from build123d import *

# Parameters (mm, degrees)
SKETCH002_W  = 7.7
SKETCH002_H  = 9.35
PAD_DEPTH    = 1
SKETCH003_W  = 7.7
SKETCH003_H  = 9.35
PAD001_DEPTH = 2.5
SKETCH004_W  = 7.7
SKETCH004_H  = 9.35
PAD002_DEPTH = 1.8
SKETCH005_R  = 3.5
PAD003_DEPTH = 5
SKETCH006_R  = 3.000001
PAD004_DEPTH = 3
PAD005_DEPTH = 7


with BuildPart() as part:
    # Sketch002 (on DatumPlane) → Pad (new body)
    with BuildSketch(Plane.XY):
        with Locations((0, -0.825)):
            Rectangle(SKETCH002_W, SKETCH002_H)
    extrude(amount=PAD_DEPTH)

    # Sketch003 (on DatumPlane) → Pad001 (join)
    with BuildSketch(Plane.XY.offset(1)):
        with Locations((0, -0.825)):
            Rectangle(SKETCH003_W, SKETCH003_H)
    extrude(amount=PAD001_DEPTH)

    # Sketch004 (on DatumPlane) → Pad002 (join)
    with BuildSketch(Plane.XY.offset(3.5)):
        with Locations((0, -0.825)):
            Rectangle(SKETCH004_W, SKETCH004_H)
    extrude(amount=PAD002_DEPTH)

    # Sketch005 (on DatumPlane) → Pad003 (join)
    with BuildSketch(Plane.XY.offset(5.3)):
        Circle(SKETCH005_R)
    extrude(amount=PAD003_DEPTH)

    # Sketch006 (on DatumPlane) → Pad004 (join)
    with BuildSketch(Plane.XY.offset(10.3)):
        Circle(SKETCH006_R)
    extrude(amount=PAD004_DEPTH)

    # Sketch007 (on DatumPlane) → Pad005 (join)
    with BuildSketch(Plane.XY.offset(13.3)):
        with BuildLine():
            ThreePointArc((-1.500001, 2.598077), (-1.500001, -2.598077), (3.000001, -1e-06))
            Line((-1.500001, 2.598077), (3.000001, -1e-06))
        make_face()
    extrude(amount=PAD005_DEPTH)


solid = part.part
For this review, take the finished solid that the model builds, in its own axes (mm). A direction names the side the tool comes from. Coordinates: 2 decimals unless noted, no trailing zeros. Loops run counter-clockwise (first coordinate to the right, second up) from the corner with the lowest first, then second, coordinate; pieces in that order, holes last. Notation, with made-up numbers: (48, 70) - (105, 70) arc R23 cw to (105, 90) - close; hole circle Ø10 at (63.25, -20). An arc over 180 degrees is marked (long way). Return JSON: item names as keys, results as strings.
Item 1: Take a section at D-D (y = -0.5). Give the boundary of the cut face in (x, z).
Determined:
{"outline": "(-3.85, 0) - (3.85, 0) - (3.85, 5.3) - (3.46, 5.3) - (3.46, 10.3) - (2.96, 10.3) - (2.96, 20.3) - (-2.96, 20.3) - (-2.96, 10.3) - (-3.46, 10.3) - (-3.46, 5.3) - (-3.85, 5.3) - close"}
Item 2: For line 1 (Z direction, x = 3.25, y = 0.5); line 2 (Z direction, x = -0.75, y = -4.25); line 3 (Y direction, x = -2, z = 19), list the stretches that pass through material, from the lowest coordinate up.
Determined:
{"line 1": "z = 0 to 10.3", "line 2": "z = 0 to 5.3", "line 3": "y = -2.24 to 2.24"}
Item 3: Take a section at B-B (z = 10). Give the boundary of the cut face in (x, y).
Determined:
{"outline": "circle Ø7 at (0, 0)"}
Item 4: For faces 1 (the flat face through (0.718, 1.317, 16.751)), 2 (the flat face through (3, 1, 10.3)), 3 (the flat face through (3.85, -1, 3)), list the 3-axis set-ups (+Z, -Z, +X, -X, +Y, -Y) from which the entire face can be reached by the end or side of a thin tool; tool diameter is ignored.
Determined:
{"face 1": "+Z, +X, +Y", "face 2": "+Z", "face 3": "+Z, -Z, +X, +Y, -Y"}
Item 5: Take a section at C-C (x = -1). Give the boundary of the cut face in (y, z), then the cut area to 3 significant figures.
Determined:
{"outline": "(-5.5, 0) - (3.85, 0) - (3.85, 5.3) - (3.35, 5.3) - (3.35, 10.3) - (2.83, 10.3) - (2.83, 13.3) - (2.31, 13.3) - (2.31, 20.3) - (-2.83, 20.3) - (-2.83, 10.3) - (-3.35, 10.3) - (-3.35, 5.3) - (-5.5, 5.3) - close", "area": "136 mm2"}
Item 6: Take a section at A-A (y = 0.5). Give the boundary of the cut face in (x, z), then the cut area to 3 significant figures.
Determined:
{"outline": "(-3.85, 0) - (3.85, 0) - (3.85, 5.3) - (3.46, 5.3) - (3.46, 10.3) - (2.96, 10.3) - (2.96, 13.3) - (2.13, 13.3) - (2.13, 20.3) - (-2.96, 20.3) - (-2.96, 10.3) - (-3.46, 10.3) - (-3.46, 5.3) - (-3.85, 5.3) - close", "area": "129 mm2"}
Item 7: Insertion check: pin 1 (1.5 mm diameter, centred on y = -3, z = 17, fed in from +X); pin 2 (3 mm diameter, centred on x = -2, z = 14.5, fed in from +Y); pin 3 (3 mm diameter, centred on x = 1.5, z = 13, fed in from +Y). Each pin has a flat end and moves straight along its axis. Give the tip position at first contact, or say it passes through.
Determined:
{"pin 1": "stops at x = 1.98", "pin 2": "stops at y = 2.79", "pin 3": "stops at y = 3"}
